```python
from build123d import *

# Parameters (mm, degrees)
BOSS_EXTRUDE1_START = -35
BOSS_EXTRUDE1_DEPTH = 70
CUT_EXTRUDE1_DEPTH  = 61.466933282
FILLET1_R           = 8


# Read off the part's stored shape, not the designer's step: Boss-Extrude1
with BuildPart() as part:
    # Boss-Extrude1 outline → Boss-Extrude1 (new body)
    with BuildSketch(Plane.XY.offset(BOSS_EXTRUDE1_START)):
        with BuildLine():
            Line((25, 34.641016151), (25, 37.382028889))
            add(Edge.make_bspline(
                [(25, 37.382028889), (23.499149868, 38.038900322), (20.42020332, 39.233525172), (12.247727699, 41.641473317), (0, 43.149082804), (-12.247727699, 41.641473317), (-20.42020332, 39.233525172), (-23.499149868, 38.038900322), (-25, 37.382028889)],
                knots=[1.070195568, 1.070195568, 1.070195568, 1.070195568, 1.168370339, 1.266545109, 1.570796327, 1.875047544, 1.973222315, 2.071397085, 2.071397085, 2.071397085, 2.071397085], degree=3))
            Line((-25, 37.382028889), (-25, 34.641016151))
            add(Edge.make_bspline(
                [(25, 34.641016151), (0, 46.188021535), (-25, 34.641016151)],
                knots=[1.047197551, 1.047197551, 1.047197551, 2.094395102, 2.094395102, 2.094395102], degree=2, weights=[1, 0.866025404, 1]))
        make_face()
    extrude(amount=BOSS_EXTRUDE1_DEPTH)

    # Sketch5 → Cut-Extrude1 (cut, through all)
    with BuildSketch(Plane(origin=(0, 0, 0), x_dir=(1, 0, 0), z_dir=(0, 1, 0))):
        with BuildLine():
            Line((-22.5, -31), (-22.5, -21))
            ThreePointArc((-22.5, -21), (-21, -19.5), (-19.5, -21))
            Line((-19.5, -21), (-19.5, -31))
            ThreePointArc((-19.5, -31), (-21, -32.5), (-22.5, -31))
        make_face()
    extrude(amount=CUT_EXTRUDE1_DEPTH, mode=Mode.SUBTRACT)

    # Fillet1
    # the kernel refuses this fillet: 8 mm, written as the material it takes off along each edge
    with BuildSketch(Plane(origin=(-25, 57.382028889, -35), x_dir=(1, 0, 0), z_dir=(0, -1, 0)), Plane(origin=(25, 14.641016151, 35), x_dir=(0, 0, -1), z_dir=(0, 1, 0))) as fillet1_piece_1:
        with BuildLine():
            CenterArc((FILLET1_R, FILLET1_R), FILLET1_R, 180, 90)
            Line((0, FILLET1_R), (0, 0))
            Line((0, 0), (FILLET1_R, 0))
        make_face()
    extrude(amount=42.741012738, mode=Mode.SUBTRACT)
    with BuildSketch(Plane(origin=(-25, 57.382028889, 35), x_dir=(1, 0, 0), z_dir=(0, -1, 0)), Plane(origin=(25, 14.641016151, -35), x_dir=(0, 0, 1), z_dir=(0, 1, 0))) as fillet1_piece_2:
        with BuildLine():
            CenterArc((FILLET1_R, -FILLET1_R), FILLET1_R, 90, 90)
            Line((0, -FILLET1_R), (0, 0))
            Line((0, 0), (FILLET1_R, 0))
        make_face()
    extrude(amount=42.741012738, mode=Mode.SUBTRACT)


solid = part.part
```
Can you work these out from the model? Positions are in its coordinate system, mm. A direction names the side the tool comes from. Give positions to 0.01 mm unless a question says otherwise; leave off trailing zeros. Write item = value, one per line. Start each with the question number.
Q1. For faces 1 (the cylindrical face through (-21, 37.6, 32.5)), 2 (the flat face through (-0.2, 40.4, -35)), which set-ups out of +Z, -Z, +X, -X, +Y, -Y let a thin tool reach every point of the face, with its end or its side?
Q2. I need wall thicknesses on probe 1 along X at (y, z) = (35.5, -3); probe 2 along Y at (x, z) = (0.5, -24); probe 3 along Y at (x, z) = (9, -30.5). Which ranges of each line are inside material? Lowest first, please. Write a range as [from, to].
Q3. Will these pins go through, and if not, where does the flat tip stop? pin 1 Ø1.5 at (x, z) = (-2.5, 4) entering from +Y; pin 2 Ø10 at (x, z) = (16.5, -24) entering from +Y; pin 3 Ø4 at (x, y) = (4, 36.5) entering from -Z; pin 4 Ø10 at (x, z) = (-12.5, 26) entering from -Y.
Q4. We'd pull the mould along Z, two halves only. Please class faces 3 (the cylindrical face through (-22.594, 37.467, 32.719)), 4 (the cylindrical face through (-21, 37.6, 19.5)), 5 (the cylindrical face through (-22.719, 36.847, -32.594)): pulls with the +Z half, pulls with the -Z half, needs draft (parallel to the pull), parting line crosses it, or undercut.
Check result:
q1.face_1 = +Y, -Y
q1.face_2 = -Z, +X, -X, +Y, -Y
q2.probe_1 = [-25, -23.04], [23.04, 25]
q2.probe_2 = [40, 42.5]
q2.probe_3 = [39.35, 41.87]
q3.pin_1 = 42.48
q3.pin_2 = 41.47
q3.pin_3 = through
q3.pin_4 = 37.47
q4.face_3 = pulls with the +Z half
q4.face_4 = undercut
q4.face_5 = pulls with the -Z half
